from build123d import *

# Parameters (mm, degrees)
SKETCH2_R           = 4.75
BOSS_EXTRUDE1_DEPTH = 6.3
SKETCH3_R           = 3.125
BOSS_EXTRUDE2_DEPTH = 50
CUT_EXTRUDE1_DEPTH  = 4.25


with BuildPart() as part:
    # Sketch2 → Boss-Extrude1 (new body)
    with BuildSketch(Plane(origin=(0, 0, 0), x_dir=(1, 0, 0), z_dir=(0, 1, 0))):
        Circle(SKETCH2_R)
    extrude(amount=BOSS_EXTRUDE1_DEPTH)

    # Sketch3 → Boss-Extrude2 (add)
    with BuildSketch(Plane.XZ):
        Circle(SKETCH3_R)
    extrude(amount=BOSS_EXTRUDE2_DEPTH)

    # Sketch4 → Cut-Extrude1 (cut)
    with BuildSketch(Plane(origin=(0, 6.3, 0), x_dir=(1, 0, 0), z_dir=(0, 1, 0))):
        Polygon((-2.4, 1.385640646), (-2.4, -1.385640646), (0, -2.771281292), (2.4, -1.385640646), (2.4, 1.385640646), (0, 2.771281292), align=None)
    extrude(amount=-CUT_EXTRUDE1_DEPTH, mode=Mode.SUBTRACT)


solid = part.part
Input: part model. Units: mm. Frame: model coordinates. A direction names the side the tool comes from. Coordinates: 2 decimals unless noted, no trailing zeros. Order: outer loops, then holes, each group sorted by start corner. A loop starts at its lowest first (then second) coordinate and runs counter-clockwise, first axis right, second up. Notation, with made-up numbers: M -31.75,-24.5 L -27.75,-24.5 A8 ccw -27.75,-15.5 Z; hole C 31,65 d7. An arc over 180 degrees is marked long. One line per question, with ' | ' between items.
Item 1: Section B-B (x = 0.75). Output: boundary loops of the cut face in (y, z), then the cut area to 3 significant figures.
Geometry results:
outline: M -50,-3.03 L 0,-3.03 L 0,-4.69 L 6.3,-4.69 L 6.3,-2.34 L 2.05,-2.34 L 2.05,2.34 L 6.3,2.34 L 6.3,4.69 L 0,4.69 L 0,3.03 L -50,3.03 Z | area: 343 mm^2
Item 2: Ray query, line 1 along X through (y, z) = (-20.5, 0.25); line 2 along Y through (x, z) = (1.75, 4); line 3 along Y through (x, z) = (0.5, -0.75). Return the intervals inside material, ascending.
Geometry results:
line 1: x = -3.11 to 3.11 | line 2: y = 0 to 6.3 | line 3: y = -50 to 2.05
Item 3: Section C-C (y = -2.5). Output: boundary loops of the cut face in (x, z) (3 decimals), then the cut area to 3 significant figures.
Geometry results:
outline: C 0,0 d6.25 | area: 30.7 mm^2
Item 4: Section A-A (z = 0). Output: boundary loops of the cut face in (x, y) (3 decimals).
Geometry results:
outline: M -4.75,0 L -3.125,0 L -3.125,-50 L 3.125,-50 L 3.125,0 L 4.75,0 L 4.75,6.3 L 2.4,6.3 L 2.4,2.05 L -2.4,2.05 L -2.4,6.3 L -4.75,6.3 Z
Item 5: Pin query (flat end, axial travel): pin 1 (5 mm diameter, centred on x = -2, y = -39, fed in from -Z) (3 decimals); pin 2 (1.4 mm diameter, centred on x = 0, z = -1, fed in from +Y); pin 3 (1 mm diameter, centred on y = -12.5, z = 1.5, fed in from +X). Return the tip coordinate at first contact, or that it passes through.
Geometry results:
pin 1: stops at z = -3.125 | pin 2: stops at y = 2.05 | pin 3: stops at x = 2.96
Item 6: Reachability of faces 1 (the flat face through (0, -50, 0)), 2 (the flat face through (1.18, 4.2, 2.09)), 3 (the cylindrical face through (2.98, -24.65, 0.94)) from +Z, -Z, +X, -X, +Y, -Y: full face, straight path, thin tool, end or side. Return the list, or none.
Geometry results:
face 1: +Z, -Z, +X, -X, -Y | face 2: +Y | face 3: -Y
Item 7: Draft query along Z for faces 4 (the flat face through (-1.217, 4.205, 2.069)), 5 (the cylindrical face through (2.192, 3.106, 4.214)), 6 (the flat face through (3.1, 0, -1.1)). Return one class per face: released by +Z, released by -Z, zero draft, split by the parting line, or undercut.
Geometry results:
face 4: undercut | face 5: split by the parting line | face 6: zero draft
